```python
from build123d import *

# Parameters (mm, degrees)
F1_DEPTH     = 30
F2_R         = 1.75
F3_DEPTH     = 16.501
F4_R         = 3
F5_DEPTH     = 13
F6_R         = 3
F7_DEPTH     = 13
F9_DEPTH     = 5
F10_T1_DEPTH = 15
F10_T3_DEPTH = 35


# Not quite as in the source:
# - a fillet or chamfer that OpenCascade refuses, or shapes differently, is made with other operations: its cross-section is extruded or revolved along the edge and cut away or added


with BuildPart() as f1:
    # F0 (on Top) → F1 (new body)
    with BuildSketch(Plane.XY):
        Polygon((0, -7.5), (0, 0), (-15, 0), (-15, -20), (0, -20), (0, -12.5), (1.5, -12.5), (1.5, -7.5), align=None)
    extrude(amount=F1_DEPTH)

    # F2 (on face) → F3 (cut, through all)
    with BuildSketch(Plane(origin=(-15, 0, 0), x_dir=(0, -1, 0), z_dir=(-1, 0, 0))):
        with Locations((10, 24)):
            Circle(F2_R)
        with Locations((10, 6)):
            Circle(F2_R)
    extrude(amount=-F3_DEPTH, mode=Mode.SUBTRACT)

    # F4 (on face) → F5 (cut)
    with BuildSketch(Plane.YZ):
        with Locations((-16.25, 15)):
            Circle(F4_R)
    extrude(amount=-F5_DEPTH, mode=Mode.SUBTRACT)

    # F6 (on face) → F7 (cut)
    with BuildSketch(Plane.YZ):
        with Locations((-3.75, 15)):
            Circle(F6_R)
    extrude(amount=-F7_DEPTH, mode=Mode.SUBTRACT)

    # F8 (on face) → F9 (join)
    with BuildSketch(Plane(origin=(0, 0, 0), x_dir=(-1, 0, 0), z_dir=(0, 1, 0))):
        Polygon((60, 30), (15, 30), (-6, 30), (0, 20), (15, 20), align=None)
    extrude(amount=F9_DEPTH)

    # F10: fillet of radius 2 on 2 edges, made by hand

    # F10_s2 → F10_t1 (join)
    with BuildSketch(Plane.YZ.offset(-15)):
        with BuildLine():
            ThreePointArc((0, 18), (0.5857864376, 19.4142135624), (2, 20))
            Line((2, 20), (0, 20))
            Line((0, 20), (0, 18))
        make_face()
    extrude(amount=F10_T1_DEPTH)

    # F10_s4 → F10_t3 (cut)
    with BuildSketch(Plane.YZ.offset(-30)):
        with BuildLine():
            ThreePointArc((5, 22), (4.4142135624, 20.5857864376), (3, 20))
            Line((3, 20), (5, 20))
            Line((5, 20), (5, 22))
        make_face()
    extrude(amount=F10_T3_DEPTH, mode=Mode.SUBTRACT)


solid = f1.part
```
Part model, mm, in its own coordinate system. A direction names the side the tool comes from. Coordinates: 2 decimals unless noted, no trailing zeros. Write each loop counter-clockwise with the first axis right and the second up, starting at its lowest first coordinate (ties: lowest second). Pieces come first, ordered by that corner, then holes.
Item 1: Pin check, flat tips, straight feed: pin 1 (1.5 mm diameter, centred on y = -10, z = 6.5, fed in from +X); pin 2 (5 mm diameter, centred on y = -15, z = 13, fed in from -X); pin 3 (1.8 mm diameter, centred on y = -17, z = 15.5, fed in from +X); pin 4 (8 mm diameter, centred on x = -2, z = 14.5, fed in from +Y). Stop position of each tip, or through.
Item 2: Slice it at B-B (y = -10). Write the cut outline in (x, z), and give its area (4 significant figures).
Item 3: Probe line 1 (Z direction, x = -3, y = -10); line 2 (Z direction, x = -8.75, y = -16.25); line 3 (Z direction, x = -3, y = -8.5). List the from-to ranges inside material, lowest first.
Item 4: Slice it at A-A (z = 6). Write the cut outline in (x, y), and give its area (3 significant figures).
Item 5: Mould opens along Z. For faces 4 (the face through (-37.18, 2.46, 24.93)), 5 (the face through (-6.866, -9.772, 25.735)), 6 (the face through (1.5, -10, 15)) say: released by +Z, released by -Z, zero draft, split by the parting line, or undercut.
Item 6: Slice it at C-C (y = -16.25). Write the cut outline in (x, z).
Item 7: Which spindle directions (+Z, -Z, +X, -X, +Y, -Y) get a long thin tool onto all of the face, cutting with end or side? Do faces 1 (the face through (0, -19.6, 14.8)), 2 (the face through (-6.41, -16.9, 12.07)), 3 (the face through (-7, 0, 9)). Say none if no direction does.
Item 8: Slice it at D-D (z = 11.25). Write the cut outline in (x, y).
Results found:
1. pin 1: passes through
1. pin 2: stops at x = -15
1. pin 3: stops at x = -13
1. pin 4: stops at y = 0.06
2. outline: (-15, 0) - (1.5, 0) - (1.5, 4.25) - (-15, 4.25) - close; (-15, 7.75) - (1.5, 7.75) - (1.5, 22.25) - (-15, 22.25) - close; (-15, 25.75) - (1.5, 25.75) - (1.5, 30) - (-15, 30) - close
2. area: 379.5 mm2
3. line 1: z = 0 to 4.25, 7.75 to 22.25, 25.75 to 30
3. line 2: z = 0 to 12, 18 to 30
3. line 3: z = 0 to 5.1, 6.9 to 23.1, 24.9 to 30
4. outline: (-15, -20) - (0, -20) - (0, -12.5) - (1.5, -12.5) - (1.5, -11.75) - (-15, -11.75) - close; (-15, -8.25) - (1.5, -8.25) - (1.5, -7.5) - (0, -7.5) - (0, 0) - (-15, 0) - close
4. area: 250 mm2
5. face 4: released by -Z
5. face 5: undercut
5. face 6: zero draft
6. outline: (-15, 0) - (0, 0) - (0, 12) - (-13, 12) - (-13, 18) - (0, 18) - (0, 30) - (-15, 30) - close
7. face 1: +Z, -Z, +X, -Y
7. face 2: +X
7. face 3: -Z, +X, -X, +Y
8. outline: (-15, -20) - (0, -20) - (0, -12.5) - (1.5, -12.5) - (1.5, -7.5) - (0, -7.5) - (0, 0) - (-15, 0) - close
